Input: dimensioned drawing with shaded views. Units: mm. Origin: part minimum x, y, z. Round coordinates to 2 decimals unless told otherwise and drop trailing zeros. Order: outer loops, then holes, each group sorted by start corner. A loop starts at its lowest first (then second) coordinate and runs counter-clockwise, first axis right, second up.
Item 1: First-contact query: pin 1 (2 mm diameter, centred on y = 1, z = 3.5, fed in from -X); pin 2 (1.5 mm diameter, centred on x = 3, z = 3.5, fed in from -Y). Flat tips, straight axial feed; report the tip coordinate or a pass-through.
Item 2: Cut plane A-A on y = 4. Output: boundary loops of the cut face in (x, z), then the cut area to 3 significant figures.
Item 3: Line query: L1, parallel to Y at x = 4, z = 1.75; L2, parallel to X at y = 5.5, z = 2.55; L3, parallel to Y at x = 5.75, z = 0.8. Output: solid intervals per line, ascending.
Item 4: Cut plane C-C on z = 0.7. Output: boundary loops of the cut face in (x, y), then the cut area to 3 significant figures.
Item 5: Cut plane D-D on z = 3.1. Output: boundary loops of the cut face in (x, y).
Item 6: Mould query, pull axis Y, two halves, no side actions, for the marked faces 1, 2 and 3. Classes: released by +Y, released by -Y, zero draft, split by the parting line, or undercut.
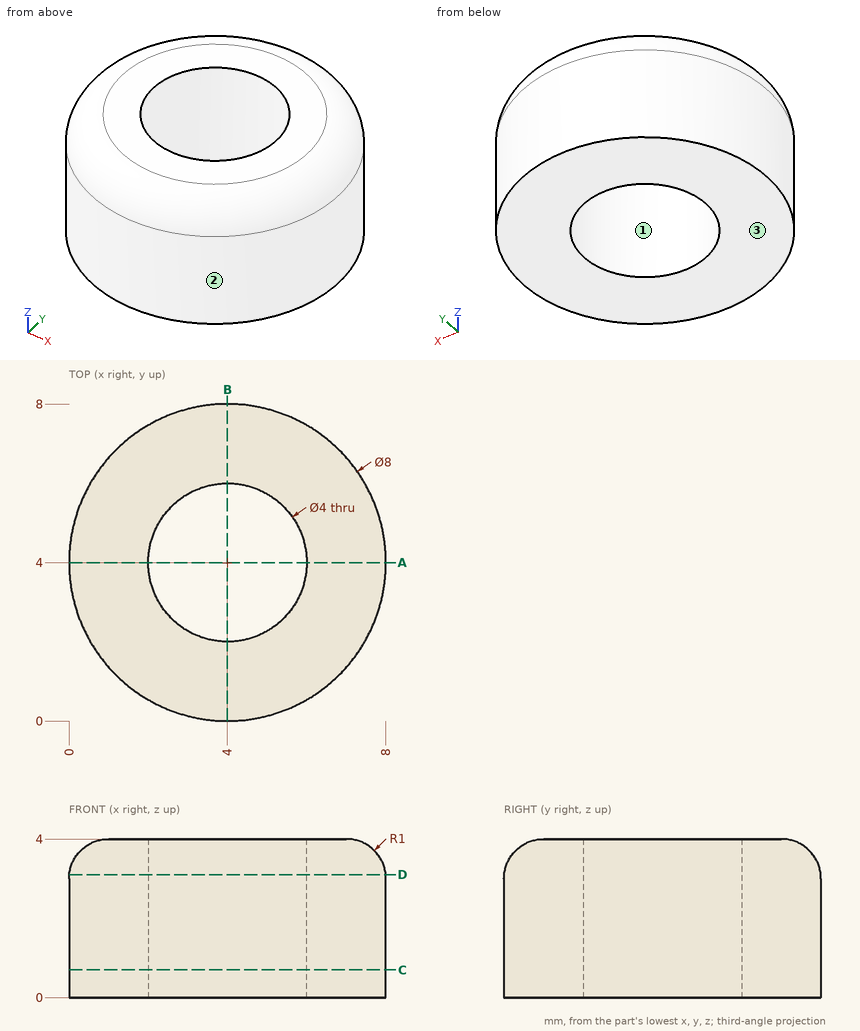
From the geometry:
1. pin 1: stops at x = 0.59
1. pin 2: stops at y = 0.02
2. outline: (0, 0) - (2, 0) - (2, 4) - (1, 4) arc R1 ccw to (0, 3) - close; (6, 0) - (8, 0) - (8, 3) arc R1 ccw to (7, 4) - (6, 4) - close
2. area: 15.6 mm2
3. L1: y = 0 to 2, 6 to 8
3. L2: x = 0.29 to 2.68, 5.32 to 7.71
3. L3: y = 0.4 to 3.03, 4.97 to 7.6
4. outline: circle Ø8 at (4, 4); hole circle Ø4 at (4, 4)
4. area: 37.7 mm2
5. outline: circle Ø7.99 at (4, 4); hole circle Ø4 at (4, 4)
6. face 1: undercut
6. face 2: split by the parting line
6. face 3: zero draft
